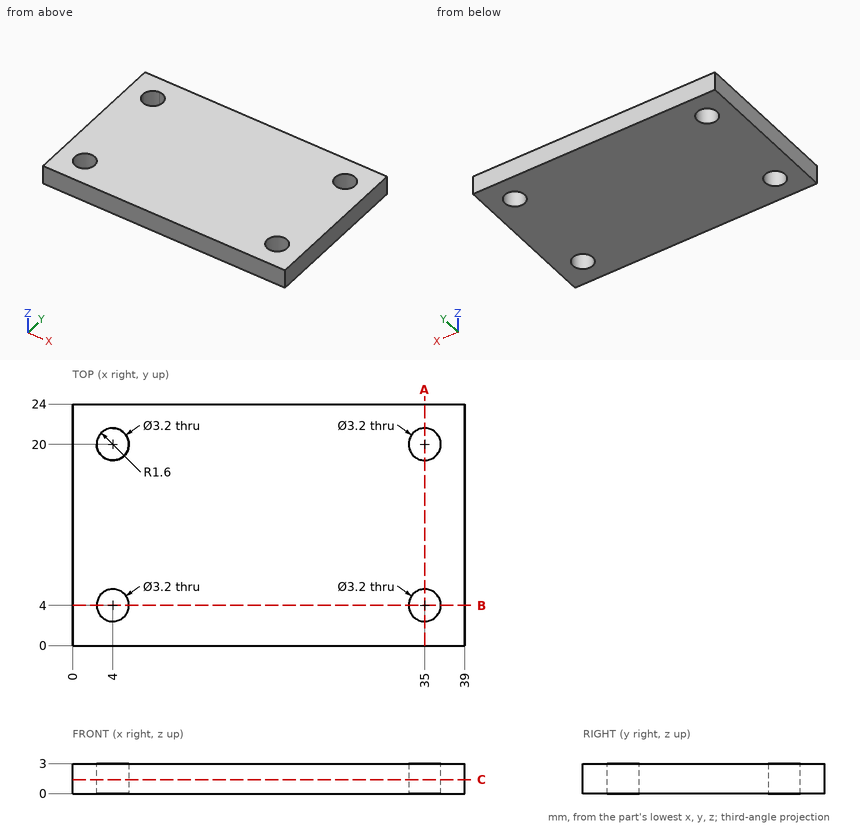
Can you work these out from the drawing? Everything is in mm from the part's minimum corner. Coordinates: 2 decimals unless noted, no trailing zeros. Write each loop counter-clockwise with the first axis right and the second up, starting at its lowest first coordinate (ties: lowest second). Pieces come first, ordered by that corner, then holes. Notation, with made-up numbers: (73.5, -13.5) -> (86.5, -13.5) arc R24 ccw to (86.5, 22.5) -> close; hole circle Ø7 at (31.5, -10). An arc over 180 degrees is marked (long way). Write item = value, one per line.
(1) Imagine slicing it at C-C (z = 1.4). Please give me the cut outline in (x, y).
Verdict:
outline = (0, 0) -> (39, 0) -> (39, 24) -> (0, 24) -> close; hole circle Ø3.2 at (4, 4); hole circle Ø3.2 at (4, 20); hole circle Ø3.2 at (35, 4); hole circle Ø3.2 at (35, 20)
(2) Imagine slicing it at A-A (x = 35). Please give me the cut outline in (y, z), and give its area (3 significant figures).
Verdict:
outline = (0, 0) -> (2.4, 0) -> (2.4, 3) -> (0, 3) -> close; (5.6, 0) -> (18.4, 0) -> (18.4, 3) -> (5.6, 3) -> close; (21.6, 0) -> (24, 0) -> (24, 3) -> (21.6, 3) -> close
area = 52.8 mm^2
(3) For pin 1 (3 mm diameter, centred on x = 4, y = 4, fed in from -Z), with a flat end and sliding along its axis, tell me the tip position at first contact or that it passes through.
Verdict:
pin_1 = through
(4) Imagine slicing it at B-B (y = 4). Please give me the cut outline in (x, z).
Verdict:
outline = (0, 0) -> (2.4, 0) -> (2.4, 3) -> (0, 3) -> close; (5.6, 0) -> (33.4, 0) -> (33.4, 3) -> (5.6, 3) -> close; (36.6, 0) -> (39, 0) -> (39, 3) -> (36.6, 3) -> close
(5) If I drill on probe 1 along Y at (x, z) = (35, 2.35), over which ranges is the centre line in solid material (lowest first)?
Verdict:
probe_1 = 0 to 2.4, 5.6 to 18.4, 21.6 to 24
